Could you check a few things on this model? Use its own coordinates, in mm. A direction names the side the tool comes from. Coordinates: 2 decimals unless noted, no trailing zeros. Write each loop counter-clockwise with the first axis right and the second up, starting at its lowest first coordinate (ties: lowest second). Pieces come first, ordered by that corner, then holes.
Item 1: For P1, Ø1, axis at x = 1, y = -0.5, coming from the +Z side, with a flat end and sliding along its axis, tell me the tip position at first contact or that it passes through.
Item 2: If I drill on probe 1 along X at (y, z) = (-0.2, -27); probe 2 along X at (y, z) = (0.1, 11.5); probe 3 along Y at (x, z) = (0.15, -25), over which ranges is the centre line in solid material (lowest first)?
Item 3: I want a section at C-C on z = 16. Please give me the cut outline in (x, y), then the cut area to 3 significant figures.
Item 4: I want a section at D-D on z = -61. Please give me the cut outline in (x, y), then the cut area to 3 significant figures.
Item 5: Which directions (+Z, -Z, +X, -X, +Y, -Y) give clear straight access to the entire face, cutting with the end or side of a thin tool? Please do faces 1 (the cylindrical face through (-0.47, -0.9, -49.3)), 2 (the cylindrical face through (0, -2, 14)).
Item 6: I want a section at A-A on x = 0. Please give me the cut outline in (y, z).
from build123d import *

# Parameters (mm, degrees)
SKETCH1_R           = 2
BOSS_EXTRUDE1_DEPTH = 30
FILLET1_R           = 2
SKETCH2_R           = 1.014585346
BOSS_EXTRUDE2_DEPTH = 100


with BuildPart() as part:
    # Sketch1 → Boss-Extrude1 (new body)
    with BuildSketch(Plane.XY):
        Circle(SKETCH1_R)
    extrude(amount=BOSS_EXTRUDE1_DEPTH)

    # Fillet1
    fillet1_edges = [part.edges().sort_by_distance(p)[0] for p in [
        (-2, 0, 30),
    ]]
    fillet(fillet1_edges, radius=FILLET1_R)

    # Sketch2 → Boss-Extrude2 (add)
    with BuildSketch(Plane(origin=(0, 0, 0), x_dir=(-1, 0, 0), z_dir=(0, 0, -1))):
        Circle(SKETCH2_R)
    extrude(amount=BOSS_EXTRUDE2_DEPTH)


solid = part.part
Response values:
1. P1: stops at z = 29.9
2. probe 1: x = -0.99 to 0.99
2. probe 2: x = -2 to 2
2. probe 3: y = -1 to 1
3. outline: circle Ø4 at (0, 0)
3. area: 12.6 mm2
4. outline: circle Ø2.03 at (0, 0)
4. area: 3.23 mm2
5. face 1: -Z
5. face 2: +Z, -Z
6. outline: (-2, 0) - (-1.01, 0) - (-1.01, -100) - (1.01, -100) - (1.01, 0) - (2, 0) - (2, 28) arc R2 ccw to (-2, 28) - close
